from build123d import *

# Parameters (mm, degrees)
SKETCH1_W           = 62.5
SKETCH1_H           = 70
BOSS_EXTRUDE1_DEPTH = 15
SKETCH2_R           = 12.5
BOSS_EXTRUDE2_DEPTH = 4
CHAMFER1_SIZE       = 2
SKETCH3_R           = 1
CUT_EXTRUDE1_DEPTH  = 10
SKETCH4_W           = 10
SKETCH4_H           = 10
CUT_EXTRUDE2_DEPTH  = 10
SKETCH5_W           = 9
SKETCH5_H           = 10
CUT_EXTRUDE3_DEPTH  = 10


with BuildPart() as part:
    # Sketch1 → Boss-Extrude1 (new, symmetric)
    with BuildSketch(Plane.XY):
        Rectangle(SKETCH1_W, SKETCH1_H)
    extrude(amount=BOSS_EXTRUDE1_DEPTH, both=True)

    # Sketch2 → Boss-Extrude2 (add, symmetric)
    with BuildSketch(Plane(origin=(0, 35, 0), x_dir=(1, 0, 0), z_dir=(0, 1, 0))):
        Circle(SKETCH2_R)
    extrude(amount=BOSS_EXTRUDE2_DEPTH, both=True)

    # Chamfer1
    chamfer1_edges = [part.edges().sort_by_distance(p)[0] for p in [
        (31.25, 0, 15),
        (0, 35, 15),
        (-31.25, 0, 15),
        (0, 35, -15),
        (31.25, 0, -15),
        (0, -35, -15),
        (-31.25, 0, -15),
        (-31.25, 35, 0),
        (31.25, 35, 0),
        (31.25, -35, 0),
        (-31.25, -35, 0),
        (0, -35, 15),
    ]]
    chamfer(chamfer1_edges, length=CHAMFER1_SIZE)

    # Sketch3 → Cut-Extrude1 (cut)
    with BuildSketch(Plane(origin=(0, 0, -15), x_dir=(-1, 0, 0), z_dir=(0, 0, -1))):
        with Locations((-24.25, 28)):
            Circle(SKETCH3_R)
        with Locations((24.25, 28)):
            Circle(SKETCH3_R)
        with Locations((-24.25, -28)):
            Circle(SKETCH3_R)
        with Locations((24.25, -28)):
            Circle(SKETCH3_R)
    extrude(amount=-CUT_EXTRUDE1_DEPTH, mode=Mode.SUBTRACT)

    # Sketch4 → Cut-Extrude2 (cut)
    with BuildSketch(Plane.XY.offset(15)):
        Rectangle(SKETCH4_W, SKETCH4_H)
    extrude(amount=-CUT_EXTRUDE2_DEPTH, mode=Mode.SUBTRACT)

    # Sketch5 → Cut-Extrude3 (cut)
    with BuildSketch(Plane(origin=(0, 0, -15), x_dir=(-1, 0, 0), z_dir=(0, 0, -1))):
        with Locations((5.5, 0)):
            Rectangle(SKETCH5_W, SKETCH5_H)
        with Locations((-5.5, 0)):
            Rectangle(SKETCH5_W, SKETCH5_H)
    extrude(amount=-CUT_EXTRUDE3_DEPTH, mode=Mode.SUBTRACT)


solid = part.part
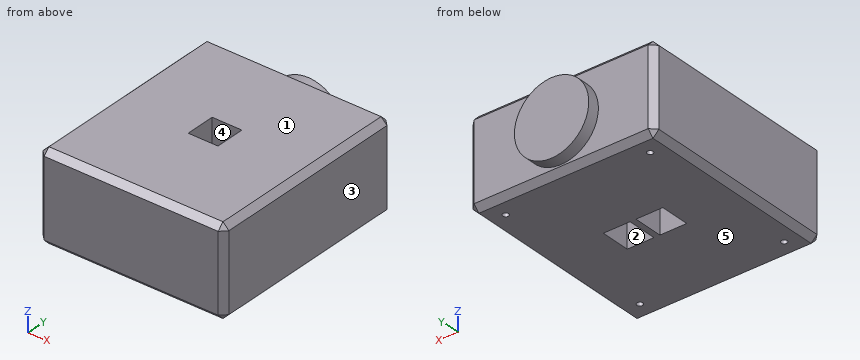
Design review of the part built by this model. Coordinates are the model's own, in mm. Face numbers are marked on the shaded views. A direction names the side the tool comes from. Give positions to 0.01 mm unless a question says otherwise; leave off trailing zeros. Loops run counter-clockwise (first coordinate to the right, second up) from the corner with the lowest first, then second, coordinate; pieces in that order, holes last. Notation, with made-up numbers: M -31.5,-20.5 L 25.5,-20.5 A11 cw 25.5,-6.5 Z; hole C -32,36.25 d8. An arc over 180 degrees is marked long. Write item = value, one per line.
Q1. We need section D-D (y = -28). Give the boundary of the cut face in (x, z), plus the area to 3 significant figures.
Output values:
outline = M -31.25,-13 L -29.25,-15 L -25.25,-15 L -25.25,-5 L -23.25,-5 L -23.25,-15 L 23.25,-15 L 23.25,-5 L 25.25,-5 L 25.25,-15 L 29.25,-15 L 31.25,-13 L 31.25,13 L 29.25,15 L -29.25,15 L -31.25,13 Z
area = 1,830 mm^2
Q2. Insertion check: pin 1 (1.6 mm diameter, centred on x = 24.25, y = 28, fed in from -Z); pin 2 (3 mm diameter, centred on x = 2, y = -0.5, fed in from +Z); pin 3 (1.5 mm diameter, centred on x = -25, z = 0.5, fed in from +Y). Each pin has a flat end and moves straight along its axis. Give the tip position at first contact, or say it passes through.
Output values:
pin_1 = -5
pin_2 = 5
pin_3 = 35
Q3. We need section A-A (z = -10). Give the boundary of the cut face in (x, y), plus the area to 3 significant figures.
Output values:
outline = M -31.25,-33 L -29.25,-35 L 29.25,-35 L 31.25,-33 L 31.25,33 L 29.25,35 L 7.5,35 L 7.5,39 L -7.5,39 L -7.5,35 L -29.25,35 L -31.25,33 Z; hole C -24.25,-28 d2; hole C -24.25,28 d2; hole M -10,-5 L -1,-5 L -1,5 L -10,5 Z; hole M 1,-5 L 10,-5 L 10,5 L 1,5 Z; hole C 24.25,-28 d2; hole C 24.25,28 d2
area = 4,230 mm^2
Q4. We need section C-C (z = 0). Give the boundary of the cut face in (x, y).
Output values:
outline = M -31.25,-33 L -29.25,-35 L 29.25,-35 L 31.25,-33 L 31.25,33 L 29.25,35 L 12.5,35 L 12.5,39 L -12.5,39 L -12.5,35 L -29.25,35 L -31.25,33 Z
Q5. For the marked faces 1 and 2, list the 3-axis set-ups (+Z, -Z, +X, -X, +Y, -Y) from which the entire face can be reached by the end or side of a thin tool; tool diameter is ignored.
Output values:
face_1 = +Z, +X, -X, +Y, -Y
face_2 = -Z
Q6. To check wall thickness, follow line 1 (Y direction, x = 24.25, z = -7); line 2 (Y direction, x = 2, z = 7); line 3 (Y direction, x = -24, z = 1.5). State the ranges of each line that lie inside material, in increasing order. Write a range as [from, to].
Output values:
line_1 = [-35, -29], [-27, 27], [29, 35]
line_2 = [-35, -5], [5, 39]
line_3 = [-35, 35]
Q7. We need section B-B (x = 0). Give the boundary of the cut face in (y, z), plus the area to 3 significant figures.
Output values:
outline = M -35,-13 L -33,-15 L 33,-15 L 35,-13 L 35,-12.5 L 39,-12.5 L 39,12.5 L 35,12.5 L 35,13 L 33,15 L 5,15 L 5,5 L -5,5 L -5,15 L -33,15 L -35,13 Z
area = 2,090 mm^2
Q8. Draft analysis for pull direction X (two halves, no side actions). For the marked faces 3, 4 and 5, state which applies: +X half, -X half, draft (parallel to the pull), parting line (faces both ways), or undercut.
Output values:
face_3 = +X half
face_4 = undercut
face_5 = draft
